from build123d import *

# Parameters (mm, degrees)
SKETCH1_R                   = 39.37
BASE_EXTRUDE_DEPTH          = 6.35
SKETCH2_R                   = 31.75
BOSS_EXTRUDE1_DEPTH         = 1.016
SKETCH3_R                   = 9.525
BOSS_EXTRUDE2_DEPTH         = 63.5
CHAMFER1_SIZE               = 0.762
F_1_4_28_TAPPED_HOLE1_D     = 5.4102
F_1_4_28_TAPPED_HOLE1_DEPTH = 19.05
CHAMFER2_SIZE               = 3.048
CHAMFER2_SIZE2              = 5.279290861


with BuildPart() as part:
    # Sketch1 → Base-Extrude (new body)
    with BuildSketch(Plane.XY):
        Circle(SKETCH1_R)
    extrude(amount=BASE_EXTRUDE_DEPTH)

    # Sketch2 → Boss-Extrude1 (add)
    with BuildSketch(Plane.XY.offset(6.35)):
        Circle(SKETCH2_R)
    extrude(amount=BOSS_EXTRUDE1_DEPTH)

    # Sketch3 → Boss-Extrude2 (add)
    with BuildSketch(Plane(origin=(0, 0, 0), x_dir=(-1, 0, 0), z_dir=(0, 0, -1))):
        with Locations(Location((0, 0, 0), (0, 0, 180))):
            Circle(SKETCH3_R)
    extrude(amount=BOSS_EXTRUDE2_DEPTH)

    # Chamfer1
    chamfer1_edges = [part.edges().sort_by_distance(p)[0] for p in [
        (-9.525, 0, 0),
        (-9.525, 0, -63.5),
    ]]
    chamfer(chamfer1_edges, length=CHAMFER1_SIZE)

    # 1/4-28 Tapped Hole1
    with Locations(Plane.XY.offset(7.366)):
        with Locations((0, 0)):
            Hole(F_1_4_28_TAPPED_HOLE1_D / 2, depth=F_1_4_28_TAPPED_HOLE1_DEPTH)

    # Chamfer2
    chamfer2_edges = [part.edges().sort_by_distance(p)[0] for p in [
        (-39.37, 0, 0),
    ]]
    chamfer2_side = [part.faces().sort_by_distance(p)[0] for p in [
        (-39.37, 0, 3.175),
    ]]
    chamfer(chamfer2_edges, length=CHAMFER2_SIZE, length2=CHAMFER2_SIZE2, reference=chamfer2_side[0])


solid = part.part
Part model, mm, in its own coordinate system. A direction names the side the tool comes from. Round coordinates to 2 decimals unless told otherwise and drop trailing zeros. Loops run counter-clockwise (first coordinate to the right, second up) from the corner with the lowest first, then second, coordinate; pieces in that order, holes last. Notation, with made-up numbers: (-13, -13.75) - (39, -13.75) arc R30 ccw to (39, 23.25) - close; hole circle Ø7 at (69.25, 58). An arc over 180 degrees is marked (long way). Answer as a JSON object with one key per item and string values.
Item 1: Band-saw the part on C-C on z = -27. List the corners of the cut face in (x, y) (3 decimals), plus the area to 3 significant figures.
Output:
{"outline": "circle Ø19.05 at (0, 0)", "area": "285 mm2"}
Item 2: Wall check: L1, parallel to Z at x = 0, y = -20; L2, parallel to Y at x = 0, z = 1; L3, parallel to Y at x = 0, z = 1.25. Give the ranges that are in metal, low to high.
Output:
{"L1": "0 to 7.37", "L2": "-35.82 to -2.71, 2.71 to 35.82", "L3": "-36.26 to -2.71, 2.71 to 36.26"}
Item 3: Pull direction Y, two halves, no side cores. Call faces 1 (the face through (-2.58, 0.81, -2.29)), 2 (the face through (3, 32, 6.35)), 3 (the face through (-2.06, 9.3, -31.32)), 4 (the face through (0, 0, -11.684)): pulls with the +Y half, pulls with the -Y half, needs draft (parallel to the pull), parting line crosses it, or undercut.
Output:
{"face 1": "undercut", "face 2": "needs draft", "face 3": "parting line crosses it", "face 4": "undercut"}
Item 4: Pin check, flat tips, straight feed: pin 1 (12 mm diameter, centred on y = 6.5, z = -7.5, fed in from -X); pin 2 (12 mm diameter, centred on y = -10, z = -43, fed in from +X); pin 3 (1 mm diameter, centred on x = 31, y = -22, fed in from -Z); pin 4 (10 mm diameter, centred on x = 18.5, z = -18.5, fed in from +Y). Stop position of each tip, or through.
Output:
{"pin 1": "x = -9.51", "pin 2": "x = 8.64", "pin 3": "z = 1.98", "pin 4": "through"}
Item 5: Band-saw the part on A-A on y = 0. List the corners of the cut face in (x, z) (3 decimals).
Output:
{"outline": "(-39.37, 3.048) - (-34.091, 0) - (-10.287, 0) - (-9.525, -0.762) - (-9.525, -62.738) - (-8.763, -63.5) - (8.763, -63.5) - (9.525, -62.738) - (9.525, -0.762) - (10.287, 0) - (34.091, 0) - (39.37, 3.048) - (39.37, 6.35) - (31.75, 6.35) - (31.75, 7.366) - (2.705, 7.366) - (2.705, -11.684) - (-2.705, -11.684) - (-2.705, 7.366) - (-31.75, 7.366) - (-31.75, 6.35) - (-39.37, 6.35) - close"}
Item 6: Tool access for faces 5 (the face through (-31.24, -23.96, 4.68)), 6 (the face through (-6.883, -30.995, 6.851)), 7 (the face through (-8, -7, 0)): list every direction of +Z, -Z, +X, -X, +Y, -Y with a clear straight run to the whole face (end or side of a thin tool).
Output:
{"face 5": "+Z, -Z", "face 6": "+Z", "face 7": "-Z"}
